```python
from build123d import *

# Parameters (mm, degrees)
F0_W     = 600
F0_H     = 600
F1_DEPTH = 500
F1_TAPER = -25
F2_T     = -2.5


with BuildPart() as f1:
    # F0 (on Front) → F1 (new body)
    with BuildSketch(Plane.XZ):
        Rectangle(F0_W, F0_H)
    extrude(amount=F1_DEPTH, taper=F1_TAPER)

    # F2
    f2_openings = [f1.faces().sort_by_distance(p)[0] for p in [
        (0, -500, 0),
    ]]
    offset(amount=F2_T, openings=f2_openings, kind=Kind.INTERSECTION)


solid = f1.part
```
Input: part model. Units: mm. Frame: model coordinates. Give positions to 0.01 mm unless a question says otherwise; leave off trailing zeros.
1. Pin query (flat end, axial travel): pin 1 Ø12 at (x, y) = (243.5, -397.5) entering from +Z; pin 2 Ø10 at (y, z) = (-348.5, 326) entering from -X; pin 3 Ø4 at (x, z) = (393.5, 280.5) entering from +Y. Return the tip coordinate at first contact, or that it passes through.
Computed:
pin 1: stops at z = 488.16
pin 2: stops at x = -464.84
pin 3: stops at y = -196.22
2. Draft query along Z for faces 1 (the face through (-8, 0, 0)), 2 (the face through (-8, -2.5, 0)). Return one class per face: released by +Z, released by -Z, zero draft, split by the parting line, or undercut.
Computed:
face 1: zero draft
face 2: undercut
3. Line query: probe 1 along Z at (x, y) = (244, -194.5); probe 2 along Z at (x, y) = (156, -80); probe 3 along X at (y, z) = (-439.5, -44.5). Output: solid intervals per line, ascending.
Computed:
probe 1: z = -390.7 to -387.94, 387.94 to 390.7
probe 2: z = -337.3 to -334.55, 334.55 to 337.3
probe 3: x = -504.94 to -502.18, 502.18 to 504.94
